Check sheet for the modelled part. Datum: model origin and axes. Units: mm. Face numbers are marked on the shaded views. Round coordinates to 2 decimals unless told otherwise and drop trailing zeros. Write each loop counter-clockwise with the first axis right and the second up, starting at its lowest first coordinate (ties: lowest second). Pieces come first, ordered by that corner, then holes. Notation, with made-up numbers: (80.25, 1) - (137.25, 1) arc R20 ccw to (137.25, 36) - close; hole circle Ø5 at (13, 66). An arc over 180 degrees is marked (long way). Answer as a JSON object with one key per item and string values. Group by question number.
Item 1: Sectioned sample at B-B on y = 28.5. Record the boundary of the cut face in (x, z) (3 decimals), plus the area to 3 significant figures.
Item 2: Sectioned sample at A-A on z = 56.5. Record the boundary of the cut face in (x, y) (3 decimals), plus the area to 3 significant figures.
Item 3: Gauge pin test, flat ends, axial feed: P1, Ø2, axis at x = 16, z = 68.5, coming from the +Y side; P2, Ø5, axis at x = 13, y = 19.5, coming from the +Z side; P3, Ø5, axis at y = 4.5, z = 65.5, coming from the +X side; P4, Ø12, axis at x = -14, z = 47, coming from the -Y side. Record the tip position at first contact, or that the pin passes through.
Item 4: Sectioned sample at D-D on x = -8. Record the boundary of the cut face in (y, z).
Item 5: Release check for a two-part mould opening along X. For the marked faces 1 and 2 record: pulls with the +X half, pulls with the -X half, needs draft (parallel to the pull), parting line crosses it, or undercut.
Item 6: Thickness scan on line 1 (Z direction, x = -33, y = 20.5) (3 decimals); line 2 (X direction, y = 2.4, z = 56.5); line 3 (X direction, y = 26, z = 26) (3 decimals). Record the ranges inside material, lowest first.
Item 7: Sectioned sample at C-C on z = 30.5. Record the boundary of the cut face in (x, y) (3 decimals).
```python
from build123d import *

# Parameters (mm, degrees)
BOSS_EXTRUDE2_DEPTH             = 8.466666667
BOSS_EXTRUDE4_DEPTH             = 3.175
F_24_0_152_DIAMETER_HOLE1_D     = 3.8608
F_24_0_152_DIAMETER_HOLE1_DEPTH = 3.175
BOSS_EXTRUDE5_DEPTH             = 33.866666667
SKETCH19_W                      = 8.466666666
SKETCH19_H                      = 8.466666667
BOSS_EXTRUDE7_DEPTH             = 11.141667582
BOSS_EXTRUDE6_DEPTH             = 4.318
RIGHTPINS_DEPTH                 = 6.35
LEFTPINS_DEPTH                  = 6.35
FRONTPINS_DEPTH                 = 6.35
PINCHAMFER_SIZE                 = 0.635
CUT_EXTRUDE1_REACH              = 109.894
CUT_EXTRUDE2_REACH              = 104.372
SKETCH21_W                      = 0.508
SKETCH21_H                      = 2.54


with BuildPart() as part:
    # Sketch3 → Boss-Extrude2 (new body)
    with BuildSketch(Plane(origin=(0, 0, 0), x_dir=(1, 0, 0), z_dir=(0, 1, 0))):
        Polygon((-29.210008467, 50.211675347), (-37.676675133, 50.211675347), (-37.676675133, -85.254991405), (-29.210008467, -85.254991405), (-29.210008467, -69.696666667), (21.589991533, -69.696666667), (21.589991533, -61.23), (-29.210008467, -61.23), align=None)
    extrude(amount=BOSS_EXTRUDE2_DEPTH)

    # Sketch12 → Boss-Extrude4 (add)
    with BuildSketch(Plane(origin=(0, 0, 0), x_dir=(1, 0, 0), z_dir=(0, 1, 0))):
        with BuildLine():
            Line((-25.75, -51.77), (-29.210008467, -51.77))
            Line((-29.210008467, -51.77), (-29.210008467, -61.23))
            Line((-29.210008467, -61.23), (-25.75, -61.23))
            ThreePointArc((-25.75, -61.23), (-21.02, -56.5), (-25.75, -51.77))
        make_face()
    extrude(amount=BOSS_EXTRUDE4_DEPTH)

    # #24 (0.152) Diameter Hole1
    with Locations(Plane(origin=(0, 3.175, 0), x_dir=(1, 0, 0), z_dir=(0, 1, 0))):
        with Locations((-25.75, 56.5), (-25.75, -56.5)):
            Hole(F_24_0_152_DIAMETER_HOLE1_D / 2, depth=F_24_0_152_DIAMETER_HOLE1_DEPTH)

    # Sketch16 → Boss-Extrude5 (add)
    with BuildSketch(Plane(origin=(0, 8.466666667, 0), x_dir=(1, 0, 0), z_dir=(0, 1, 0))):
        Polygon((-37.676675133, -85.254991405), (-37.676675133, -52.64717283), (-31.115008467, -52.64717283), (-31.115008467, 41.74500868), (-37.676675133, 41.74500868), (-37.676675133, 50.211675347), (-29.210008467, 50.211675347), (-29.210008467, -85.254991405), align=None)
    extrude(amount=BOSS_EXTRUDE5_DEPTH)

    # Sketch19 → Boss-Extrude7 (add)
    with BuildSketch(Plane(origin=(0, 8.466666667, 0), x_dir=(1, 0, 0), z_dir=(0, 1, 0))):
        with Locations((17.3566582, -65.463333334)):
            Rectangle(SKETCH19_W, SKETCH19_H)
    extrude(amount=BOSS_EXTRUDE7_DEPTH)

    # Sketch18 → Boss-Extrude6 (add)
    with BuildSketch(Plane(origin=(0, 0, 61.23), x_dir=(-1, 0, 0), z_dir=(0, 0, -1))):
        Polygon((-21.589991533, 19.608334249), (29.210008467, 42.333333333), (29.210008467, 8.466666667), (-13.123324867, 8.466666667), (-13.123324867, 19.608334249), align=None)
    extrude(amount=-BOSS_EXTRUDE6_DEPTH)

    # Sketch4 → RightPins (cut)
    with BuildSketch(Plane.XY.offset(85.254991405)):
        Polygon((-36.6183418, 4.233333333), (-33.4433418, 7.408333333), (-30.2683418, 4.233333333), (-33.4433418, 1.058333333), align=None)
        Polygon((-36.6183418, 38.1), (-33.4433418, 41.275), (-30.2683418, 38.1), (-33.4433418, 34.925), align=None)
    extrude(amount=-RIGHTPINS_DEPTH, mode=Mode.SUBTRACT)

    # Sketch5 → LeftPins (cut)
    with BuildSketch(Plane(origin=(0, 0, -50.211675347), x_dir=(-1, 0, 0), z_dir=(0, 0, -1))):
        Polygon((30.2683418, 4.233333333), (33.4433418, 7.408333333), (36.6183418, 4.233333333), (33.4433418, 1.058333333), align=None)
        Polygon((30.2683418, 38.1), (33.4433418, 41.275), (36.6183418, 38.1), (33.4433418, 34.925), align=None)
    extrude(amount=-LEFTPINS_DEPTH, mode=Mode.SUBTRACT)

    # Sketch11 → FrontPins (cut)
    with BuildSketch(Plane(origin=(21.589991533, 0, 0), x_dir=(0, 0, -1), z_dir=(1, 0, 0))):
        Polygon((-68.638333333, 4.233333333), (-65.463333333, 7.408333333), (-62.288333333, 4.233333333), (-65.463333333, 1.058333333), align=None)
        Polygon((-68.638333333, 15.375000915), (-65.463333333, 18.550000915), (-62.288333333, 15.375000915), (-65.463333333, 12.200000915), align=None)
    extrude(amount=-FRONTPINS_DEPTH, mode=Mode.SUBTRACT)

    # PinChamfer
    pinchamfer_edges = [part.edges().sort_by_distance(p)[0] for p in [
        (-35.0308418, 2.645833333, 78.904991405),
        (-35.0308418, 5.820833333, 78.904991405),
        (-31.8558418, 5.820833333, 78.904991405),
        (-31.8558418, 2.645833333, 78.904991405),
        (-35.0308418, 2.645833333, 85.254991405),
        (-31.8558418, 2.645833333, 85.254991405),
        (-31.8558418, 5.820833333, 85.254991405),
        (-35.0308418, 5.820833333, 85.254991405),
        (-35.0308418, 36.5125, 78.904991405),
        (-35.0308418, 39.6875, 78.904991405),
        (-31.8558418, 39.6875, 78.904991405),
        (-31.8558418, 36.5125, 78.904991405),
        (-35.0308418, 36.5125, 85.254991405),
        (-31.8558418, 36.5125, 85.254991405),
        (-31.8558418, 39.6875, 85.254991405),
        (-35.0308418, 39.6875, 85.254991405),
        (-31.8558418, 2.645833333, -43.861675347),
        (-31.8558418, 5.820833333, -43.861675347),
        (-35.0308418, 5.820833333, -43.861675347),
        (-35.0308418, 2.645833333, -43.861675347),
        (-31.8558418, 2.645833333, -50.211675347),
        (-35.0308418, 2.645833333, -50.211675347),
        (-35.0308418, 5.820833333, -50.211675347),
        (-31.8558418, 5.820833333, -50.211675347),
        (-31.8558418, 36.5125, -43.861675347),
        (-31.8558418, 39.6875, -43.861675347),
        (-35.0308418, 39.6875, -43.861675347),
        (-35.0308418, 36.5125, -43.861675347),
        (-31.8558418, 36.5125, -50.211675347),
        (-35.0308418, 36.5125, -50.211675347),
        (-35.0308418, 39.6875, -50.211675347),
        (-31.8558418, 39.6875, -50.211675347),
        (15.239991533, 2.645833333, 67.050833333),
        (15.239991533, 5.820833333, 67.050833333),
        (15.239991533, 5.820833333, 63.875833333),
        (15.239991533, 2.645833333, 63.875833333),
        (21.589991533, 2.645833333, 67.050833333),
        (21.589991533, 2.645833333, 63.875833333),
        (21.589991533, 5.820833333, 63.875833333),
        (21.589991533, 5.820833333, 67.050833333),
        (15.239991533, 13.787500915, 67.050833333),
        (15.239991533, 16.962500915, 67.050833333),
        (15.239991533, 16.962500915, 63.875833333),
        (15.239991533, 13.787500915, 63.875833333),
        (21.589991533, 13.787500915, 67.050833333),
        (21.589991533, 13.787500915, 63.875833333),
        (21.589991533, 16.962500915, 63.875833333),
        (21.589991533, 16.962500915, 67.050833333),
    ]]
    chamfer(pinchamfer_edges, length=PINCHAMFER_SIZE)

    # Sketch20 → Cut-Extrude1 (cut, up to next)
    with BuildSketch(Plane(origin=(-29.210008467, 0, 0), x_dir=(0, 0, -1), z_dir=(1, 0, 0)), mode=Mode.PRIVATE) as cut_extrude1_sk1:
        with BuildLine():
            Line((41.74500868, 25.4), (41.74500868, 42.333333333))
            Line((41.74500868, 42.333333333), (29.04500868, 42.333333333))
            Line((29.04500868, 42.333333333), (29.04500868, 25.4))
            ThreePointArc((29.04500868, 25.4), (35.39500868, 19.05), (41.74500868, 25.4))
        make_face()
    cut_extrude1_tool1 = extrude(cut_extrude1_sk1.sketch, amount=-CUT_EXTRUDE1_REACH, mode=Mode.PRIVATE) & part.part
    add(cut_extrude1_tool1.solids().sort_by_distance((-29.210008, 31.327209, -35.395009))[0], mode=Mode.SUBTRACT)

    # Sketch21 → Cut-Extrude2 (cut, up to next)
    with BuildSketch(Plane(origin=(0, 42.333333333, 0), x_dir=(1, 0, 0), z_dir=(0, 1, 0)), mode=Mode.PRIVATE) as cut_extrude2_sk1:
        with Locations((-37.422675133, 48.179675347)):
            Rectangle(SKETCH21_W, SKETCH21_H)
    cut_extrude2_tool1 = extrude(cut_extrude2_sk1.sketch, amount=-CUT_EXTRUDE2_REACH, mode=Mode.PRIVATE) & part.part
    add(cut_extrude2_tool1.solids().sort_by_distance((-37.422675, 42.333333, -48.179675))[0], mode=Mode.SUBTRACT)


solid = part.part
```
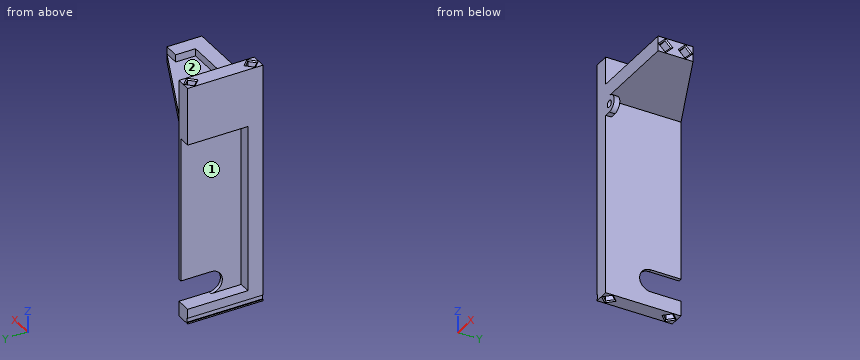
Completed:
{
 "1": {"outline": "(-37.677, -50.212) - (-29.21, -50.212) - (-29.21, -41.745) - (-37.677, -41.745) - (-37.677, -46.91) - (-37.169, -46.91) - (-37.169, -49.45) - (-37.677, -49.45) - close; (-37.677, 52.647) - (-31.115, 52.647) - (-31.115, -29.045) - (-29.21, -29.045) - (-29.21, 61.23) - (1.713, 61.23) - (1.713, 65.548) - (-29.21, 65.548) - (-29.21, 85.255) - (-37.677, 85.255) - close", "area": "636 mm²"},
 "2": {"outline": "(-37.677, 0) - (-27.68, 0) - (-27.68, 3.175) - (-29.21, 3.175) - (-29.21, 42.333) - (-37.677, 42.333) - close; (-23.82, 0) - (-21.02, 0) - (-21.02, 3.175) - (-23.82, 3.175) - close", "area": "372 mm²"},
 "3": {"P1": "y = 19.61", "P2": "z = 69.7", "P3": "x = 21.42", "P4": "through"},
 "4": {"outline": "(0, 61.23) - (32.85, 61.23) - (32.85, 65.55) - (8.47, 65.55) - (8.47, 69.7) - (0, 69.7) - close"},
 "5": {"face 1": "pulls with the -X half", "face 2": "undercut"},
 "6": {"line 1": "-50.212 to -41.745, 52.647 to 85.255", "line 2": "-37.68 to -27.68, -23.82 to -21.02", "line 3": "-31.115 to -29.21"},
 "7": {"outline": "(-37.677, 0) - (-29.21, 0) - (-29.21, 42.333) - (-31.115, 42.333) - (-31.115, 8.467) - (-37.677, 8.467) - close"}
}
